For this review, take the finished solid that the model builds, in its own axes (mm). Face numbers are marked on the shaded views. A direction names the side the tool comes from. Give positions to 0.01 mm unless a question says otherwise; leave off trailing zeros. Loops run counter-clockwise (first coordinate to the right, second up) from the corner with the lowest first, then second, coordinate; pieces in that order, holes last.
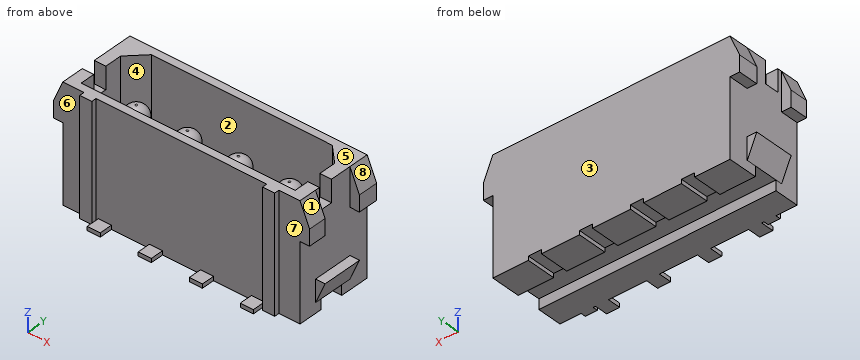
```python
from build123d import *

# Parameters (mm, degrees)
BOSS_EXTRUDE1_DEPTH = 4.15
SKETCH2_W           = 10
SKETCH2_H           = 5
SKETCH2_W_2         = 17
CUT_EXTRUDE1_DEPTH  = 12.5
SKETCH3_W           = 5
SKETCH3_H           = 4
CUT_EXTRUDE2_DEPTH  = 6.3
SKETCH4_W           = 5
SKETCH4_H           = 4.540427611
SKETCH4_H_2         = 5
CUT_EXTRUDE3_DEPTH  = 6.3
CUT_EXTRUDE4_DEPTH  = 7.3
SKETCH6_R           = 1.11
BOSS_EXTRUDE2_DEPTH = 5.1
FILLET1_R           = 1
SKETCH7_W           = 5
SKETCH7_H           = 1.4
CUT_EXTRUDE5_DEPTH  = 25.55
SKETCH8_W           = 1.3
SKETCH8_H           = 3
CUT_EXTRUDE6_DEPTH  = 9.3
SKETCH9_W           = 3
SKETCH9_H           = 2.4
CUT_EXTRUDE7_DEPTH  = 25.55
SKETCH10_W          = 1.3
SKETCH10_H          = 0.4
BOSS_EXTRUDE3_DEPTH = 6.5
SKETCH11_W          = 20
SKETCH11_H          = 5
CUT_EXTRUDE8_DEPTH  = 12.5


with BuildPart() as part:
    # Sketch1 → Boss-Extrude1 (new body, symmetric)
    with BuildSketch(Plane(origin=(0, 0, 0), x_dir=(1, 0, 0), z_dir=(0, 1, 0))):
        Polygon((-11.8, 0), (11.8, 0), (11.8, -1), (12.75, -3.2), (11.8, -3.2), (11.8, -7.7), (12.75, -7.7), (12.75, -9.3), (11.8, -11.5), (-11.8, -11.5), (-12.75, -9.3), (-12.75, -7.7), (-11.8, -7.7), (-11.8, -3.2), (-12.75, -3.2), (-11.8, -1), align=None)
    extrude(amount=BOSS_EXTRUDE1_DEPTH, both=True)

    # Sketch2 → Cut-Extrude1 (cut, through all)
    with BuildSketch(Plane.XY.offset(11.5)):
        with Locations((14.7, -6.15)):
            Rectangle(SKETCH2_W, SKETCH2_H)
        with Locations((-14.7, -6.15)):
            Rectangle(SKETCH2_W, SKETCH2_H)
        with Locations((0, -6.15)):
            Rectangle(SKETCH2_W_2, SKETCH2_H)
    extrude(amount=-CUT_EXTRUDE1_DEPTH, mode=Mode.SUBTRACT)

    # Sketch3 → Cut-Extrude2 (cut)
    with BuildSketch(Plane.XY.offset(11.5)):
        with Locations((14.3, 0.15)):
            Rectangle(SKETCH3_W, SKETCH3_H)
        with Locations((-14.3, 0.15)):
            Rectangle(SKETCH3_W, SKETCH3_H)
    extrude(amount=-CUT_EXTRUDE2_DEPTH, mode=Mode.SUBTRACT)

    # Sketch4 → Cut-Extrude3 (cut)
    with BuildSketch(Plane(origin=(0, 0, 0), x_dir=(-1, 0, 0), z_dir=(0, 0, -1))):
        with Locations((14.3, 4.420213806)):
            Rectangle(SKETCH4_W, SKETCH4_H)
        with Locations((14.3, -4.35)):
            Rectangle(SKETCH4_W, SKETCH4_H_2)
        with Locations((-14.3, -4.35)):
            Rectangle(SKETCH4_W, SKETCH4_H_2)
        with Locations((-14.3, 4.65)):
            Rectangle(SKETCH4_W, SKETCH4_H_2)
    extrude(amount=-CUT_EXTRUDE3_DEPTH, mode=Mode.SUBTRACT)

    # Sketch5 → Cut-Extrude4 (cut)
    with BuildSketch(Plane.XY.offset(11.5)):
        Polygon((-10.65, -2.875), (10.65, -2.875), (10.65, 1.725), (9, 3.375), (-9, 3.375), (-10.65, 1.725), align=None)
    extrude(amount=-CUT_EXTRUDE4_DEPTH, mode=Mode.SUBTRACT)

    # Sketch6 → Boss-Extrude2 (add)
    with BuildSketch(Plane.XY.offset(4.2)):
        with Locations((-7.62, 0)):
            Circle(SKETCH6_R)
        with Locations((-2.54, 0)):
            Circle(SKETCH6_R)
        with Locations((2.54, -3.41e-07)):
            Circle(SKETCH6_R)
        with Locations((7.62, 0)):
            Circle(SKETCH6_R)
    extrude(amount=BOSS_EXTRUDE2_DEPTH)

    # Fillet1
    fillet1_edges = [part.edges().sort_by_distance(p)[0] for p in [
        (-8.73, 0, 9.3),
        (-3.65, 0, 9.3),
        (1.43, -3.41e-07, 9.3),
        (6.51, 0, 9.3),
    ]]
    fillet(fillet1_edges, radius=FILLET1_R)

    # Sketch7 → Cut-Extrude5 (cut, through all)
    with BuildSketch(Plane(origin=(11.8, 0, 0), x_dir=(0, 0, -1), z_dir=(1, 0, 0))):
        with Locations((-11.8, -0.7)):
            Rectangle(SKETCH7_W, SKETCH7_H)
    extrude(amount=-CUT_EXTRUDE5_DEPTH, mode=Mode.SUBTRACT)

    # Sketch8 → Cut-Extrude6 (cut, through all)
    with BuildSketch(Plane(origin=(0, 4.15, 0), x_dir=(1, 0, 0), z_dir=(0, 1, 0))):
        with Locations((-7.62, 1.1)):
            Rectangle(SKETCH8_W, SKETCH8_H)
        with Locations((-2.54, 1.1)):
            Rectangle(SKETCH8_W, SKETCH8_H)
        with Locations((2.54, 1.1)):
            Rectangle(SKETCH8_W, SKETCH8_H)
        with Locations((7.62, 1.1)):
            Rectangle(SKETCH8_W, SKETCH8_H)
    extrude(amount=-CUT_EXTRUDE6_DEPTH, mode=Mode.SUBTRACT)

    # Sketch9 → Cut-Extrude7 (cut, through all)
    with BuildSketch(Plane(origin=(11.8, 0, 0), x_dir=(0, 0, -1), z_dir=(1, 0, 0))):
        with Locations((0.5, 0)):
            Rectangle(SKETCH9_W, SKETCH9_H)
    extrude(amount=-CUT_EXTRUDE7_DEPTH, mode=Mode.SUBTRACT)

    # Sketch10 → Boss-Extrude3 (add)
    with BuildSketch(Plane(origin=(0, -1.2, 0), x_dir=(1, 0, 0), z_dir=(0, 1, 0))):
        with Locations((-7.62, -0.2)):
            Rectangle(SKETCH10_W, SKETCH10_H)
        with Locations((-2.54, -0.2)):
            Rectangle(SKETCH10_W, SKETCH10_H)
        with Locations((2.54, -0.2)):
            Rectangle(SKETCH10_W, SKETCH10_H)
        with Locations((7.62, -0.2)):
            Rectangle(SKETCH10_W, SKETCH10_H)
    extrude(amount=-BOSS_EXTRUDE3_DEPTH)

    # Sketch11 → Cut-Extrude8 (cut, through all)
    with BuildSketch(Plane(origin=(0, 0, 0), x_dir=(-1, 0, 0), z_dir=(0, 0, -1))):
        with Locations((0, -7.45)):
            Rectangle(SKETCH11_W, SKETCH11_H)
    extrude(amount=-CUT_EXTRUDE8_DEPTH, mode=Mode.SUBTRACT)


solid = part.part
```
Item 1: Clearance check with flat-ended pins moving along their axes: pin 1 Ø1 at (x, y) = (-2.5, -4.5) entering from +Z; pin 2 Ø1.5 at (x, z) = (1, 2.5) entering from -Y; pin 3 Ø0.6 at (x, y) = (11.5, -0.5) entering from +Z. State where each tip first meets the part, or that it passes through.
Answer:
pin 1: stops at z = 0.4
pin 2: stops at y = -3.65
pin 3: stops at z = 9.3
Item 2: Take a section at A-A on z = 5.5. Give the boundary of the cut face in (x, y) (3 decimals).
Answer:
outline: (-11.8, -3.65) - (-9.7, -3.65) - (-9.7, -4.15) - (-8.5, -4.15) - (-8.5, -3.65) - (8.5, -3.65) - (8.5, -4.15) - (9.7, -4.15) - (9.7, -3.65) - (11.8, -3.65) - (11.8, 4.15) - (-11.8, 4.15) - close; circle Ø2.22 at (-7.62, 0); circle Ø2.22 at (-2.54, 0); circle Ø2.22 at (2.54, 0); circle Ø2.22 at (7.62, 0); hole (-10.65, -2.875) - (10.65, -2.875) - (10.65, 1.725) - (9, 3.375) - (-9, 3.375) - (-10.65, 1.725) - close
Item 3: Take a section at C-C on x = -10. Give the boundary of the cut face in (y, z) (3 decimals), and give its area (3 significant figures).
Answer:
outline: (-3.65, 0) - (-1.2, 0) - (-1.2, 1) - (1.2, 1) - (1.2, 0) - (4.15, 0) - (4.15, 11.5) - (2.375, 11.5) - (2.375, 4.2) - (-2.875, 4.2) - (-2.875, 11.5) - (-3.65, 11.5) - close
area: 49.0 mm2
Item 4: Take a section at B-B on z = 1.25. Give the boundary of the cut face in (x, y), and give its area (3 significant figures).
Answer:
outline: (-11.91, -1.85) - (-11.8, -1.85) - (-11.8, -3.65) - (-9.7, -3.65) - (-9.7, -4.15) - (-8.5, -4.15) - (-8.5, -3.65) - (8.5, -3.65) - (8.5, -4.15) - (9.7, -4.15) - (9.7, -3.65) - (11.8, -3.65) - (11.8, -1.85) - (11.91, -1.85) - (11.91, 2.15) - (11.8, 2.15) - (11.8, 4.15) - (-11.8, 4.15) - (-11.8, 2.15) - (-11.91, 2.15) - close
area: 186 mm2
Item 5: Tool access review of the marked faces 4, 5, 6, 7 and 8: name each direction out of +Z, -Z, +X, -X, +Y, -Y from which nothing blocks a thin tool from reaching the whole face with its end or side.
Answer:
face 4: +Z
face 5: +Z, +X, -X, +Y, -Y
face 6: +Z, -Z, -X, -Y
face 7: +Z, -Z, +X, -Y
face 8: +Z, +X, +Y, -Y
Item 6: For L1, parallel to Y at x = -0.25, z = 8 (3 decimals); L2, parallel to X at y = -1.25, z = 8.5; L3, parallel to X at y = 1, z = 6.25, list the stretches that pass through material, from the lowest coordinate up.
Answer:
L1: y = -3.65 to -2.875, 3.375 to 4.15
L2: x = -11.8 to -10.65, 10.65 to 11.8
L3: x = -11.8 to -10.65, -8.1 to -7.14, -3.02 to -2.06, 2.06 to 3.02, 7.14 to 8.1, 10.65 to 11.8
Item 7: The part is to be moulded in two halves that separate along X. For the marked faces 1, 2 and 3, say which applies: released by +X, released by -X, zero draft, split by the parting line, or undercut.
Answer:
face 1: released by +X
face 2: undercut
face 3: zero draft
